Read the model definition and answer for the solid it produces. Units are mm, in the model's axes. Give positions to 0.01 mm unless a question says otherwise; leave off trailing zeros. Order: outer loops, then holes, each group sorted by start corner. A loop starts at its lowest first (then second) coordinate and runs counter-clockwise, first axis right, second up. Notation, with made-up numbers: (84, 53.25) - (128, 53.25) arc R19 cw to (128, 70.25) - close; hole circle Ø8 at (-6, -11.5). An arc over 180 degrees is marked (long way). Use a Markdown table: item, result. Add a question column.
1. Consider L1, parallel to Z at x = 25.25, y = 7.5; L2, parallel to Y at x = 0.8, z = -14; L3, parallel to X at y = 6, z = 54. Determine where each line is inside the solid, lowest interval first.
2. A cutting plane is placed at A-A on z = 26.5. Determine the outline of the cut face in (x, y).
3. Flat-ended cylindrical pins translate along their axes: P1, Ø8.5, axis at x = 16.5, z = 142, coming from the +Y side; P2, Ø1, axis at y = 13, z = 122.5, coming from the +X side. Find the tip coordinate at first contact, or state that the pin passes through.
```python
from build123d import *

# Parameters (mm, degrees)
BOSS_EXTRUDE1_DEPTH      = 410
BOSS_EXTRUDE1_DEPTH_BACK = 20
F_3_0_3_DIAMETER_HOLE1_D = 3
F_3_0_3_DIAMETER_HOLE2_D = 3
F_3_0_3_DIAMETER_HOLE3_D = 3
F_3_0_3_DIAMETER_HOLE4_D = 3


with BuildPart() as part:
    # Sketch1 → Boss-Extrude1 (new, two sides: drawn at the far end of the back side and taken through both)
    with BuildSketch(Plane.XY.offset(-BOSS_EXTRUDE1_DEPTH_BACK)):
        Polygon((0, 5.602318429), (0, 35.602318429), (2, 35.602318429), (2, 7.602318429), (30, 7.602318429), (30, 5.602318429), align=None)
    extrude(amount=BOSS_EXTRUDE1_DEPTH + BOSS_EXTRUDE1_DEPTH_BACK)

    # Ø3.0 (3) Diameter Hole1 (through all)
    with Locations(Plane(origin=(2, -3.805314364, 221.32004832), x_dir=(0, 0, -1), z_dir=(1, 0, 0))):
        with Locations((-182.67995168, 17.407632793), (-182.67995168, 31.407632793)):
            Hole(F_3_0_3_DIAMETER_HOLE1_D / 2)

    # Ø3.0 (3) Diameter Hole2 (through all)
    with Locations(Plane(origin=(2, -3.805314364, 221.32004832), x_dir=(0, 0, -1), z_dir=(1, 0, 0))):
        with Locations((235.32004832, 17.407632793), (235.32004832, 31.407632793)):
            Hole(F_3_0_3_DIAMETER_HOLE2_D / 2)

    # Ø3.0 (3) Diameter Hole3 (through all)
    with Locations(Plane(origin=(130.861996081, 5.602318429, 221.32004832), x_dir=(-1, 0, 0), z_dir=(0, -1, 0))):
        with Locations((105.861996081, -133.67995168), (120.861996081, -124.67995168), (105.861996081, -116.67995168)):
            Hole(F_3_0_3_DIAMETER_HOLE3_D / 2)

    # Ø3.0 (3) Diameter Hole4 (through all)
    with Locations(Plane(origin=(130.861996081, 5.602318429, 221.32004832), x_dir=(-1, 0, 0), z_dir=(0, -1, 0))):
        with Locations((105.861996081, 174.32004832), (105.861996081, 157.32004832), (120.861996081, 167.32004832)):
            Hole(F_3_0_3_DIAMETER_HOLE4_D / 2)


solid = part.part
```
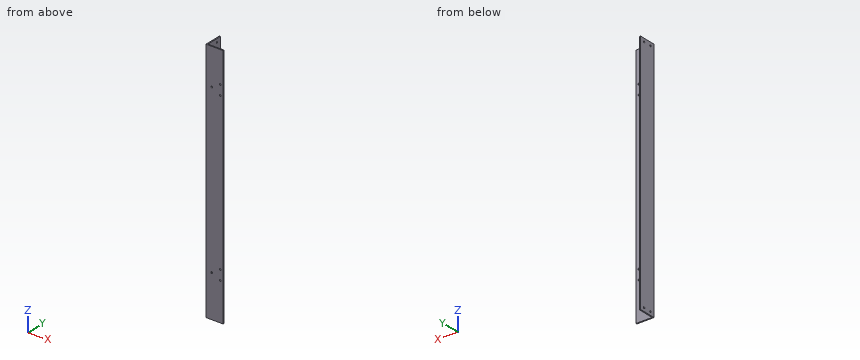
Output values:
| question | item | result |
|---|---|---|
| 1 | L1 | -20 to 45.52, 48.48 to 62.52, 65.48 to 336.52, 339.48 to 353.52, 356.48 to 410 |
| 1 | L2 | 5.6 to 12.1, 15.1 to 26.1, 29.1 to 35.6 |
| 1 | L3 | 0 to 8.5, 11.5 to 30 |
| 2 | outline | (0, 5.6) - (30, 5.6) - (30, 7.6) - (2, 7.6) - (2, 35.6) - (0, 35.6) - close |
| 3 | P1 | y = 7.6 |
| 3 | P2 | x = 2 |
